from build123d import *

# Parameters (mm, degrees)
BOSS_EXTRUDE1_DEPTH = 10
DRAFT1_ANGLE        = 20
SHELL1_T            = -3
SKETCH3_R           = 1.7
CUT_EXTRUDE1_DEPTH  = 3
CIRPATTERN1_COUNT   = 3


with BuildPart() as part:
    # Sketch2 → Boss-Extrude1 (new body)
    with BuildSketch(Plane(origin=(0, 0, 0), x_dir=(1, 0, 0), z_dir=(0, 1, 0))):
        Polygon((25.720557456, -6.800689768), (24.074489233, 11.323225041), (11.16369994, 24.148877009), (-6.970708626, 25.67500104), (-21.843445154, 15.187506739), (-26.495390933, -2.406390756), (-18.74984883, -18.874311272), (-2.231044079, -26.510731779), (15.331690993, -21.742486253), align=None)
    extrude(amount=BOSS_EXTRUDE1_DEPTH)

    # Draft1
    draft1_faces = [part.faces().sort_by_distance(p)[0] for p in [
        (-24.169418044, 5, -6.390557991),
        (-14.40707689, 5, -20.431253889),
        (2.096495657, 5, -24.911939024),
        (17.619094586, 5, -17.736051025),
        (24.897523344, 5, -2.261267636),
        (20.526124224, 5, 14.27158801),
        (-10.490446454, 5, 22.692521526),
        (-22.622619881, 5, 10.640351014),
        (6.550323457, 5, 24.126609016),
    ]]
    draft(draft1_faces, Plane.ZX.offset(10), DRAFT1_ANGLE)

    # Shell1
    shell1_openings = [part.faces().sort_by_distance(p)[0] for p in [
        (0, 0, 0),
    ]]
    offset(amount=SHELL1_T, openings=shell1_openings, kind=Kind.INTERSECTION)

    # Sketch3 → Cut-Extrude1 (cut)
    with BuildSketch(Plane(origin=(6.626174522, 9.204622905, 24.40598896), x_dir=(0.969216093, -0.086883963, -0.23037218), z_dir=(0.246211625, 0.342020143, 0.906863858))):
        with Locations((0.443378447, -4.774813723)):
            Circle(SKETCH3_R)
    cut_extrude1 = extrude(amount=-CUT_EXTRUDE1_DEPTH, mode=Mode.SUBTRACT)

    # CirPattern1: Cut-Extrude1 ×3 about axis
    cirpattern1_axis = Axis((0, 10, 0), (0, 1, 0))
    for i in range(1, CIRPATTERN1_COUNT):
        add(cut_extrude1.rotate(cirpattern1_axis, i * 360 / CIRPATTERN1_COUNT), mode=Mode.SUBTRACT)


solid = part.part
Can you work these out from the model? Positions are in its coordinate system, mm. A direction names the side the tool comes from. Coordinates: 2 decimals unless noted, no trailing zeros. Loops run counter-clockwise (first coordinate to the right, second up) from the corner with the lowest first, then second, coordinate; pieces in that order, holes last. Notation, with made-up numbers: (19, 51.5) - (41, 51.5) arc R28 cw to (41, 89.5) - close; hole circle Ø5 at (-16, 80). An arc over 180 degrees is marked (long way). Answer as a JSON object with one key per item and string values. Group by question number.
Item 1: If I drill on L1, parallel to Y at x = -12, z = 10.5; L2, parallel to X at y = 6, z = -18.5; L3, parallel to Z at x = 0, y = 4.75, over which ranges is the centre line in solid material (lowest first)? Write a range as from..to.
Item 2: If we section it at B-B (x = -3.5): List the corners of the cut face in (y, z) for me, plus the area to 3 significant figures.
Item 3: If we section it at C-C (z = 12.5): List the corners of the cut face in (x, y) for me, plus the area to 3 significant figures.
Item 4: For pin 1 (1 mm diameter, centred on y = 8.5, z = -19, fed in from +X); pin 2 (1 mm diameter, centred on x = -12.5, z = -2, fed in from -Y); pin 3 (2 mm diameter, centred on y = 6.5, z = 9.5, fed in from +X), each with a flat end and sliding along its axis, tell me the tip position at first contact or that it passes through.
Item 5: If we section it at D-D (y = 1.25): List the corners of the cut face in (x, z) for me, plus the area to 3 significant figures.
Item 6: If we section it at A-A (y = 7.75): List the corners of the cut face in (x, z) for me (3 decimals).
Item 7: If we mould it in two halves opening along X, with no side actions, what happens to faces 1 (the face through (-26.51, 4.93, -4.76)), 2 (the face through (5.4, 3.3, 25.3)), 3 (the face through (-1, 0, -26))? For each: released by +X, released by -X, zero draft, split by the parting line, or undercut.
Item 8: On a 3-axis mill with a long thin cutter (end or side, diameter ignored), from which of +Z, -Z, +X, -X, +Y, -Y can I reach the whole of each face in a straight line? I mean faces 4 (the face through (19.788, 3.451, 13.916)), 5 (the face through (26.75, 4.93, -2.28)). Say none if no direction works.
Returned:
{
 "1": {"L1": "y = 7..10", "L2": "x = -19.67..-14.13, 14.39..17.81", "L3": "z = -27.01..-23.8, 24.58..27.89"},
 "2": {"outline": "(0, -29.04) - (10, -25.38) - (10, 25.92) - (0, 29.93) - (0, 26.42) - (7, 23.61) - (7, -23.27) - (0, -25.83) - close", "area": "204 mm²"},
 "3": {"outline": "(-25.77, 0) - (-22.24, 0) - (-19.43, 7) - (19.2, 7) - (22.3, 0) - (26.19, 0) - (21.76, 10) - (-21.75, 10) - close", "area": "186 mm²"},
 "4": {"pin 1": "stops at x = 17.69", "pin 2": "stops at y = 7", "pin 3": "stops at x = 26.22"},
 "5": {"outline": "(-29.87, 2.71) - (-24.63, -17.12) - (-7.86, -28.95) - (12.59, -27.23) - (27.14, -12.77) - (29, 7.67) - (17.28, 24.51) - (-2.52, 29.89) - (-21.14, 21.28) - close; hole (-26.49, 2.41) - (-21.84, -15.18) - (-6.97, -25.67) - (11.16, -24.14) - (24.07, -11.32) - (25.71, 6.8) - (15.33, 21.74) - (-2.23, 26.5) - (-18.74, 18.87) - close", "area": "556 mm²"},
 "6": {"outline": "(-27.363, 2.485) - (-22.559, -15.685) - (-7.199, -26.516) - (11.529, -24.94) - (24.863, -11.694) - (26.563, 7.023) - (15.834, 22.455) - (-2.304, 27.379) - (-19.364, 19.493) - close"},
 "7": {"face 1": "released by -X", "face 2": "undercut", "face 3": "zero draft"},
 "8": {"face 4": "-Y", "face 5": "-Z, +X, +Y"}
}
